from build123d import *

# Parameters (mm, degrees)
F0_R     = 30
F0_R_2   = 4.25
F1_DEPTH = 10
F2_R     = 16.5
F3_DEPTH = 30
F4_W     = 12.5
F4_H     = 12.5
F5_DEPTH = 15


with BuildPart() as f1:
    # F0 (on Top) → F1 (new body)
    with BuildSketch(Plane.XY):
        Circle(F0_R)
        with Locations((-16.5, -16.51)):
            Circle(F0_R_2, mode=Mode.SUBTRACT)
        with Locations((16.5, -16.51)):
            Circle(F0_R_2, mode=Mode.SUBTRACT)
        with Locations((-16.5, 16.51)):
            Circle(F0_R_2, mode=Mode.SUBTRACT)
        with Locations((16.5, 16.51)):
            Circle(F0_R_2, mode=Mode.SUBTRACT)
    extrude(amount=F1_DEPTH)

    # F2 (on face) → F3 (join)
    with BuildSketch(Plane.XY.offset(10)):
        Circle(F2_R)
    extrude(amount=F3_DEPTH)

    # F4 (on face) → F5 (join)
    with BuildSketch(Plane.XY.offset(40)):
        Rectangle(F4_W, F4_H)
    extrude(amount=F5_DEPTH)


solid = f1.part
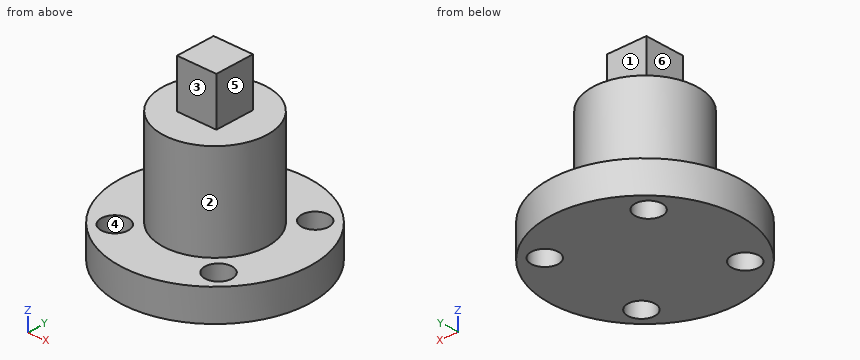
The listing builds one solid part. Answer for the finished solid, in the listing's coordinates (mm). Face numbers are marked on the shaded views. A direction names the side the tool comes from. Coordinates: 2 decimals unless noted, no trailing zeros. Order: outer loops, then holes, each group sorted by start corner. A loop starts at its lowest first (then second) coordinate and runs counter-clockwise, first axis right, second up.
Q1. A cutting plane is placed at A-A, the plane x = 0. Write down the section's boundary in (y, z), and give its area (3 significant figures).
Q2. A cutting plane is placed at C-C, the plane z = 20. Write down the section's boundary in (x, y), and give its area (3 significant figures).
Q3. A cutting plane is placed at D-D, the plane y = 8. Write down the section's boundary in (x, z), and give its area (3 significant figures).
Q4. Given P1, Ø2, axis at y = -4, z = 21, coming from the -X side (3 decimals); P2, Ø1.5, axis at y = -1.5, z = 10.5, coming from the -X side; P3, Ø1.5, axis at x = 8, z = 41, coming from the -Y side; P4, Ø1, axis at x = 8, y = 16, coming from the +Z side, each flat-ended and moving along its own axis, determine where each tip first touches the part or whether it passes through.
Q5. Which of the six approach directions +Z, -Z, +X, -X, +Y, -Y give full straight-line access (tool end or side, diameter ignored) to the marked faces 1, 2 and 3?
Q6. Consider line 1 (Y direction, x = -15, z = 4); line 2 (Y direction, x = 16.5, z = 5.25); line 3 (Z direction, x = 1, y = 26). Determine where each line is inside the solid, lowest interval first.
Q7. For a pull along X with two mould halves and no side action, classify the marked faces 4, 5 and 6 as pulls with the +X half, pulls with the -X half, needs draft (parallel to the pull), parting line crosses it, or undercut.
Answers follow:
1. outline: (-30, 0) - (30, 0) - (30, 10) - (16.5, 10) - (16.5, 40) - (6.25, 40) - (6.25, 55) - (-6.25, 55) - (-6.25, 40) - (-16.5, 40) - (-16.5, 10) - (-30, 10) - close
1. area: 1,780 mm2
2. outline: circle Ø33 at (0, 0)
2. area: 855 mm2
3. outline: (-28.91, 0) - (28.91, 0) - (28.91, 10) - (14.43, 10) - (14.43, 40) - (-14.43, 40) - (-14.43, 10) - (-28.91, 10) - close
3. area: 1,440 mm2
4. P1: stops at x = -16.225
4. P2: stops at x = -29.99
4. P3: passes through
4. P4: stops at z = 10
5. face 1: +Z, +X, -X, +Y
5. face 2: +Z
5. face 3: +Z, +X, -X, -Y
6. line 1: y = -25.98 to -20.49, -12.53 to 12.53, 20.49 to 25.98
6. line 2: y = -25.05 to -20.76, -12.26 to 12.26, 20.76 to 25.05
6. line 3: z = 0 to 10
7. face 4: undercut
7. face 5: pulls with the +X half
7. face 6: pulls with the -X half
